Autodesk Inventor part; units mm, degrees
ref_plane "YZ Plane" through (0, 0, 0) normal (1, 0, 0) x (0, 1, 0)
ref_plane "XZ Plane" through (0, 0, 0) normal (0, 1, 0) x (-1, 0, 0)
ref_plane "XY Plane" through (0, 0, 0) normal (0, 0, 1) x (1, 0, 0)
sketch "Sketch1" plane through (0, 0, 0) normal (1, 0, 0) x (0, 1, 0)
  point P0 (0, 0)
sketch "Sketch2" plane through (0, 0, 0) normal (1, 0, 0) x (0, 1, 0)
  line L0 (11.5, 16) -> (-11.5, 16)
  line L1 (-11.5, 16) -> (-11.5, -16)
  line L2 (-11.5, -16) -> (11.5, -16)
  line L3 (11.5, -16) -> (11.5, 16)
  point P0 (0, 0)
  point P1 (11.5, 0)
  point P2 (0, 16)
  dimension "d0" = 32
  dimension "d1" = 23
extrude "Extrusion1" add sketch "Sketch2" along normal blind 600
sketch "Sketch3" plane through (0, -11.5, 16) normal (0, 0, 1) x (1, 0, 0)
  line L0 (0, 23) -> (0, 0)
  line L1 (0, 0) -> (600, 0)
  line L2 (600, 23) -> (600, 0)
  line L3 (0, 23) -> (600, 23)
  line L4 (0, 23) -> (600, 23)
  circle A0 centre (25, 23) radius 8.05
  circle A1 centre (85, 23) radius 8.05
  circle A2 centre (55, 23) radius 4.5
  line L5 (300, 23) -> (300, 0) construction
  circle A3 centre (575, 23) radius 8.05
  circle A4 centre (515, 23) radius 8.05
  circle A5 centre (545, 23) radius 4.5
  point P0 (0, 11.5)
  dimension "d4" = 60
  dimension "d5" = 30
  dimension "d6" = 16.1
  dimension "d7" = 25
  dimension "d8" = 9
extrude "Extrusion2" cut sketch "Sketch3" against normal through all contours A0 L3 | L3 A0 | A2 L3 | L3 A2 | A3 L3 | L3 A3 | A1 L3 | L3 A1 | A5 L3 | L3 A5 | A4 L3 | L3 A4
sketch "Sketch4" plane through (93.05, 11.5, -16) normal (0, 1, 0) x (1, 0, 0)
  line L0 (413.9, -32) -> (413.9, 0)
  line L1 (0, 0) -> (413.9, 0)
  line L2 (0, 0) -> (0, -32)
  line L3 (0, -32) -> (413.9, -32)
  line L4 (-16.1, -32) -> (-16.1, 0)
  line L5 (-33.55, 0) -> (-16.1, 0)
  line L6 (-33.55, 0) -> (-33.55, -32)
  line L7 (-33.55, -32) -> (-16.1, -32)
  line L8 (-42.55, -32) -> (-42.55, 0)
  line L9 (-60, 0) -> (-42.55, 0)
  line L10 (-60, 0) -> (-60, -32)
  line L11 (-60, -32) -> (-42.55, -32)
  line L12 (-76.1, -32) -> (-76.1, 0)
  line L13 (-93.05, 0) -> (-76.1, 0)
  line L14 (-93.05, 0) -> (-93.05, -32)
  line L15 (-93.05, -32) -> (-76.1, -32)
  line L16 (430, 0) -> (430, -32)
  line L17 (430, -32) -> (447.45, -32)
  line L18 (447.45, -32) -> (447.45, 0)
  line L19 (430, 0) -> (447.45, 0)
  line L20 (456.45, 0) -> (456.45, -32)
  line L21 (456.45, -32) -> (473.9, -32)
  line L22 (473.9, -32) -> (473.9, 0)
  line L23 (456.45, 0) -> (473.9, 0)
  line L24 (490, 0) -> (490, -32)
  line L25 (490, -32) -> (506.95, -32)
  line L26 (506.95, 0) -> (506.95, -32)
  line L27 (490, 0) -> (506.95, 0)
  line L28 (506.95, 0) -> (506.95, -32) construction
  line L29 (506.95, -16) -> (-93.05, -16) construction
  line L30 (-93.05, 0) -> (506.95, 0) construction
  line L31 (206.95, 0) -> (206.95, -32) construction
  circle A0 centre (498.475, -16) radius 3.25
  circle A1 centre (465.175, -16) radius 3.25
  circle A2 centre (438.725, -16) radius 3.25
  circle A3 centre (206.95, -16) radius 3.25
  circle A4 centre (-24.825, -16) radius 3.25
  circle A5 centre (-51.275, -16) radius 3.25
  circle A6 centre (-84.575, -16) radius 3.25
  point P0 (438.725, 0)
  point P1 (465.175, 0)
  point P2 (498.475, 0)
  point P3 (-84.575, 0)
  point P4 (-51.275, 0)
  point P5 (-24.825, 0)
extrude "Extrusion3" cut sketch "Sketch4" against normal through all contours A0 | A1 | A2 | A3 | A4 | A5 | A6
properties part number "X_STRUCTURAL_SUP" material "Wood (Birch)"
Here's how the part is built. I have some questions about the finished solid (model axes, mm). Round coordinates to 2 decimals unless told otherwise and drop trailing zeros. Order: outer loops, then holes, each group sorted by start corner. A loop starts at its lowest first (then second) coordinate and runs counter-clockwise, first axis right, second up. Notation, with made-up numbers: M -30,-27 L -9,-27 A19 ccw -9,-19 Z; hole C -7.5,27.5 d9. An arc over 180 degrees is marked long. Answer as CSV lines item,"result".
Item 1: We'd pull the mould along X, two halves only. Please class faces 1 (the cylindrical face through (514.823, 3.452, 0.224)), 2 (the flat face through (591, 11.5, -4)), 3 (the flat face through (0, 0, 0)): +X half, -X half, draft (parallel to the pull), parting line (faces both ways), or undercut.
From the geometry:
face 1,"undercut"
face 2,"draft"
face 3,"-X half"
Item 2: For pin 1 (4 mm diameter, centred on x = 558.225, z = 0, fed in from -Y), with a flat end and sliding along its axis, tell me the tip position at first contact or that it passes through.
From the geometry:
pin 1,"through"
Item 3: Imagine slicing it at B-B on x = 575. List the corners of the cut face in (y, z) for me, and give its area (3 significant figures).
From the geometry:
outline,"M -11.5,-16 L 3.45,-16 L 3.45,16 L -11.5,16 Z"
area,"478 mm2"
Item 4: Please list where these lines run through material, in increasing order: L1, parallel to Z at x = 300, y = 6.5; L2, parallel to X at y = 4.75, z = -8; L3, parallel to X at y = 5.5, z = -8.5. Write a range as [from, to].
From the geometry:
L1,"[-16, -3.25], [3.25, 16]"
L2,"[0, 20.61], [29.39, 80.61], [89.39, 510.61], [519.39, 570.61], [579.39, 600]"
L3,"[0, 19.63], [30.37, 79.63], [90.37, 509.63], [520.37, 569.63], [580.37, 600]"
Item 5: Imagine slicing it at A-A on z = 9. List the corners of the cut face in (x, y) for me.
From the geometry:
outline,"M 0,-11.5 L 600,-11.5 L 600,11.5 L 583.05,11.5 A8.05 cw 566.95,11.5 L 549.5,11.5 A4.5 cw 540.5,11.5 L 523.05,11.5 A8.05 cw 506.95,11.5 L 93.05,11.5 A8.05 cw 76.95,11.5 L 59.5,11.5 A4.5 cw 50.5,11.5 L 33.05,11.5 A8.05 cw 16.95,11.5 L 0,11.5 Z"
